Check sheet for the modelled part. Datum: model origin and axes. Units: mm. Face numbers are marked on the shaded views. A direction names the side the tool comes from. Coordinates: 2 decimals unless noted, no trailing zeros. Loops run counter-clockwise (first coordinate to the right, second up) from the corner with the lowest first, then second, coordinate; pieces in that order, holes last.
Autodesk Inventor part; units mm, degrees
ref_plane "Work Plane1" through (0, 0, -10) normal (0, 0, 1) x (1, 0, 0)
ref_plane "YZ Plane" through (0, 0, 0) normal (1, 0, 0) x (0, 1, 0)
ref_plane "XZ Plane" through (0, 0, 0) normal (0, 1, 0) x (-1, 0, 0)
ref_plane "Work Plane1" through (0, 0, -10) normal (0, 0, 1) x (1, 0, 0)
sketch "Sketch1" plane through (0, 0, -10) normal (0, 0, 1) x (1, 0, 0)
  line L0 (0, -17.5) -> (0, 17.5) construction
  line L1 (-14, 0) -> (14, 0) construction
  line L2 (10, -7.5) -> (10, 7.5)
  arc A0 (10, 7.5) -> (-10, 7.5) centre (0, 0) ccw
  line L3 (-10, 7.5) -> (-10, -7.5)
  arc A1 (-10, -7.5) -> (10, -7.5) centre (0, 0) ccw
  circle A2 centre (0, -8) radius 1.55
  circle A3 centre (0, 8) radius 1.55
  line L4 (0, -8) -> (0, 8) construction
  line L5 (-9, -5) -> (9, -5)
  line L6 (9, -5) -> (9, 5)
  line L7 (9, 5) -> (-9, 5)
  line L8 (-9, 5) -> (-9, -5)
  line L9 (-7.5, -3) -> (7.5, -3)
  line L10 (7.5, -3) -> (7.5, 3)
  line L11 (7.5, 3) -> (-7.5, 3)
  line L12 (-7.5, 3) -> (-7.5, -3)
  line L13 (8.75, -4.75) -> (-8.75, -4.75)
  line L14 (-8.75, -4.75) -> (-8.75, 4.75)
  line L15 (-8.75, 4.75) -> (8.75, 4.75)
  line L16 (8.75, 4.75) -> (8.75, -4.75)
  point P0 (0, 0)
  point P1 (-10, 0)
  point P2 (10, 0)
  dimension "d1" = 15
  dimension "d2" = 12.5
  dimension "d3" = 20
  dimension "d4" = 3.1
  dimension "d5" = 16
  dimension "d6" = 18
  dimension "d7" = 10
  dimension "d8" = 15
  dimension "d9" = 6
  dimension "d18" = 0.25
extrude "Extrusion1" add sketch "Sketch1" along normal blind 14.7 contours A1 L3 A0 L2 | L8 L7 L6 L5 | L13 L14 L15 L16
extrude "Extrusion2" add sketch "Sketch1" along normal blind 5 from surface at 14.7 contours L13 L14 L15 L16
extrude "Extrusion3" cut sketch "Sketch1" along normal blind 4.5 contours L8 L7 L6 L5 | L13 L14 L15 L16
fillet "Fillet1" radius 1 12 edges at (-7.5, -3, 2.1) (-7.5, 3, 2.1) (7.5, 3, 2.1) (7.5, -3, 2.1) (9, -5, -7.75) (9, 5, -7.75) (-9, -5, -7.75) (-9, 5, -7.75) (-8.75, -4.75, 7.2) (-8.75, 4.75, 7.2) (8.75, -4.75, 7.2) (8.75, 4.75, 7.2)
chamfer "Chamfer1" distance 0.5 angle 45 8 edges at (9, 0, -10) (8.7071, 4.7071, -10) (0, 5, -10) (-8.7071, 4.7071, -10) (-9, 0, -10) (-8.7071, -4.7071, -10) (0, -5, -10) (8.7071, -4.7071, -10)
properties part number "Hip Adapter"
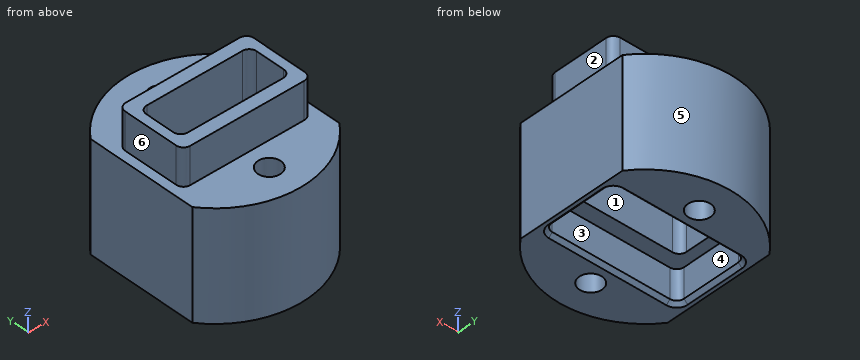
1) Depth check by flat-ended pin: pin 1 (4 mm diameter, centred on y = -9, z = -2.5, fed in from +X); pin 2 (8 mm diameter, centred on x = 4.5, z = -7.5, fed in from +Y); pin 3 (5.5 mm diameter, centred on x = 0, z = 7.5, fed in from -Y); pin 4 (4 mm diameter, centred on y = -0.5, z = 7, fed in from -X). Enter the tip coordinate at first touch or a pass-through.
Answer sheet:
pin 1: stops at x = 10
pin 2: stops at y = 12.49
pin 3: stops at y = -4.75
pin 4: stops at x = -8.75
2) Scan lines: line 1 (Y direction, x = 0, z = 0.25); line 2 (Y direction, x = 0, z = -6.75); line 3 (X direction, y = -1.5, z = 6.75). Record each from-to range of solid material in increasing order.
Answer sheet:
line 1: y = -12.5 to -9.55, -6.45 to -3, 3 to 6.45, 9.55 to 12.5
line 2: y = -12.5 to -9.55, -6.45 to -5, 5 to 6.45, 9.55 to 12.5
line 3: x = -8.75 to -7.5, 7.5 to 8.75
3) Set-up check for the marked faces 1, 2 and 3: record each of +Z, -Z, +X, -X, +Y, -Y from which the full face is reachable in a straight line by a thin tool's end or side.
Answer sheet:
face 1: +Z, -Z
face 2: +Z, +X, +Y, -Y
face 3: -Z
4) Section check D-D on x = -2. Enter the section's corners in (y, z).
Answer sheet:
outline: (-12.34, -10) - (-5.5, -10) - (-5, -9.5) - (-5, -5.5) - (-3, -5.5) - (-3, 9.7) - (-4.75, 9.7) - (-4.75, 4.7) - (-12.34, 4.7) - close; (3, -5.5) - (5, -5.5) - (5, -9.5) - (5.5, -10) - (12.34, -10) - (12.34, 4.7) - (4.75, 4.7) - (4.75, 9.7) - (3, 9.7) - close
5) Section check A-A on x = 0. Enter the section's corners in (y, z).
Answer sheet:
outline: (-12.5, -10) - (-9.55, -10) - (-9.55, 4.7) - (-12.5, 4.7) - close; (-6.45, -10) - (-5.5, -10) - (-5, -9.5) - (-5, -5.5) - (-3, -5.5) - (-3, 9.7) - (-4.75, 9.7) - (-4.75, 4.7) - (-6.45, 4.7) - close; (3, -5.5) - (5, -5.5) - (5, -9.5) - (5.5, -10) - (6.45, -10) - (6.45, 4.7) - (4.75, 4.7) - (4.75, 9.7) - (3, 9.7) - close; (9.55, -10) - (12.5, -10) - (12.5, 4.7) - (9.55, 4.7) - close
6) Mould release check, pull along Y, two halves, no side actions. Record for the marked faces 4, 5 and 6: +Y half, -Y half, draft (parallel to the pull), parting line (faces both ways), or undercut.
Answer sheet:
face 4: undercut
face 5: +Y half
face 6: draft
7) Section check C-C on y = -8. Enter the section's corners in (x, z), plus the area to 3 significant figures.
Answer sheet:
outline: (-9.6, -10) - (-1.55, -10) - (-1.55, 4.7) - (-9.6, 4.7) - close; (1.55, -10) - (9.6, -10) - (9.6, 4.7) - (1.55, 4.7) - close
area: 237 mm2
8) Section check B-B on z = -1.5. Enter the section's corners in (x, y).
Answer sheet:
outline: (-10, -7.5) arc R12.5 ccw to (10, -7.5) - (10, 7.5) arc R12.5 ccw to (-10, 7.5) - close; hole (-7.5, -2) arc R1 ccw to (-6.5, -3) - (6.5, -3) arc R1 ccw to (7.5, -2) - (7.5, 2) arc R1 ccw to (6.5, 3) - (-6.5, 3) arc R1 ccw to (-7.5, 2) - close; hole circle Ø3.1 at (0, -8); hole circle Ø3.1 at (0, 8)
